Geometry check sheet. Reference: the model listing, model coordinates, mm. Face numbers are marked on the shaded views. A direction names the side the tool comes from. Give positions to 0.01 mm unless a question says otherwise; leave off trailing zeros. Write each loop counter-clockwise with the first axis right and the second up, starting at its lowest first coordinate (ties: lowest second). Pieces come first, ordered by that corner, then holes. Notation, with made-up numbers: (-29.75, 3) -> (-12.75, 3) arc R30 ccw to (-12.75, 41) -> close; hole circle Ø5 at (19.5, 58). An arc over 180 degrees is marked (long way). Write item = value, one per line. Start each with the question number.
1. Depth check by flat-ended pin: P1, Ø5, axis at x = 67, z = -4.5, coming from the -Y side; P2, Ø20, axis at x = 71.5, z = -2, coming from the +Y side; P3, Ø2, axis at y = 31.5, z = 40.5, coming from the +X side; P4, Ø4, axis at x = 70.03, z = -10, coming from the +Y side. Enter the tip coordinate at first touch or a pass-through.
2. Set-up check for the marked faces 1, 2 and 3: record each of +Z, -Z, +X, -X, +Y, -Y from which the full face is reachable in a straight line by a thin tool's end or side.
3. Cross-section at C-C, the plane y = 21. Record the cut outline in (x, z), plus the area to 3 significant figures.
4. Cross-section at A-A, the plane z = 41.5. Record the cut outline in (x, y).
5. Cross-section at D-D, the plane z = -10. State how many separate pieces and enclosed holes the cut face has, plus the area to 3 significant figures.
6. Thickness scan on line 1 along X through (y, z) = (9, -10); line 2 along Y through (x, z) = (40.75, 10.5); line 3 along Z through (x, y) = (40.5, 36.5). Record the ranges inside material, lowest first.
7. Mould release check, pull along Y, two halves, no side actions. Record for the marked faces 4, 5 and 6: pulls with the +Y half, pulls with the -Y half, needs draft (parallel to the pull), parting line crosses it, or undercut.
8. Cross-section at B-B, the plane x = 44. Record the cut outline in (y, z), plus the area to 3 significant figures.
```python
from build123d import *

# Parameters (mm, degrees)
SKETCH1_W           = 67
SKETCH1_H           = 41.999999434
BOSS_EXTRUDE1_DEPTH = 6.000000983
SKETCH2_W           = 24.999999441
SKETCH2_H           = 29.999998398
BOSS_EXTRUDE2_DEPTH = 50
SKETCH3_W           = 19.999999553
SKETCH3_H           = 19.999999553
CUT_EXTRUDE1_DEPTH  = 85.314886613
SKETCH14_R          = 11.2
CUT_EXTRUDE12_DEPTH = 10
SKETCH15_R          = 2.6
CUT_EXTRUDE13_DEPTH = 112.961295121
SKETCH18_R          = 1.5
CUT_EXTRUDE14_DEPTH = 81.454956308
SKETCH19_R          = 2.6
CUT_EXTRUDE15_DEPTH = 113.063962124
SKETCH20_R          = 28.543107088
BOSS_EXTRUDE3_DEPTH = 5
BOSS_EXTRUDE4_REACH = 132.242
SKETCH21_W          = 30.03647221
SKETCH21_H          = 5
SKETCH22_W          = 8.074560758
SKETCH22_H          = 29.943227156
CUT_EXTRUDE16_DEPTH = 10


with BuildPart() as part:
    # Sketch1 → Boss-Extrude1 (new body)
    with BuildSketch(Plane(origin=(45.028056949, 0, 0), x_dir=(0, 0, -1), z_dir=(1, 0, 0))):
        with Locations((-13.500000447, 20.999999717)):
            Rectangle(SKETCH1_W, SKETCH1_H)
    extrude(amount=-BOSS_EXTRUDE1_DEPTH)

    # Sketch2 → Boss-Extrude2 (add)
    with BuildSketch(Plane(origin=(45.028056949, 0, 0), x_dir=(0, 0, -1), z_dir=(1, 0, 0))):
        with Locations((7.499999833, 20.999999251)):
            Rectangle(SKETCH2_W, SKETCH2_H)
    extrude(amount=BOSS_EXTRUDE2_DEPTH)

    # Sketch3 → Cut-Extrude1 (cut, through all)
    with BuildSketch(Plane.ZY.offset(-39.028055966)):
        with Locations((-9.999999777, 20.999999716)):
            Rectangle(SKETCH3_W, SKETCH3_H)
    extrude(amount=-CUT_EXTRUDE1_DEPTH, mode=Mode.SUBTRACT)

    # Sketch14 → Cut-Extrude12 (cut)
    with BuildSketch(Plane(origin=(45.028056949, 0, 0), x_dir=(0, 0, -1), z_dir=(1, 0, 0))):
        with Locations((-25.999999888, 20.999999251)):
            Circle(SKETCH14_R)
    extrude(amount=-CUT_EXTRUDE12_DEPTH, mode=Mode.SUBTRACT)

    # Sketch15 → Cut-Extrude13 (cut, through all)
    with BuildSketch(Plane(origin=(0, 6.000000052, 0), x_dir=(-1, 0, 0), z_dir=(0, -1, 0))):
        with Locations(Location((-50.028056949, 9.999999553, 0), (0, 0, 90))):
            Circle(SKETCH15_R)
        with Locations(Location((-70.028056949, 9.999999553, 0), (0, 0, 90))):
            Circle(SKETCH15_R)
    extrude(amount=-CUT_EXTRUDE13_DEPTH, mode=Mode.SUBTRACT)

    # Sketch18 → Cut-Extrude14 (cut, through all)
    with BuildSketch(Plane(origin=(45.028056949, 0, 0), x_dir=(0, 0, -1), z_dir=(1, 0, 0))):
        with Locations((-10.499999888, 36.499999251)):
            Circle(SKETCH18_R)
        with Locations((-10.499999888, 5.499999251)):
            Circle(SKETCH18_R)
        with Locations((-41.499999888, 5.499999251)):
            Circle(SKETCH18_R)
        with Locations((-41.499999888, 36.499999251)):
            Circle(SKETCH18_R)
    extrude(amount=-CUT_EXTRUDE14_DEPTH, mode=Mode.SUBTRACT)

    # Sketch19 → Cut-Extrude15 (cut, through all)
    with BuildSketch(Plane.XY.offset(4.999999888)):
        with Locations((70.028056949, 20.999999251)):
            Circle(SKETCH19_R)
    extrude(amount=-CUT_EXTRUDE15_DEPTH, mode=Mode.SUBTRACT)

    # Sketch20 → Boss-Extrude3 (add)
    with BuildSketch(Plane(origin=(95.028056949, 0, 0), x_dir=(0, 0, -1), z_dir=(1, 0, 0))):
        with Locations(Location((-6.802134848, 21.140269153, 0), (0, 0, 327.965134835))):
            Circle(SKETCH20_R)
    extrude(amount=BOSS_EXTRUDE3_DEPTH)

    # Sketch21 → Boss-Extrude4 (add, up to next)
    with BuildSketch(Plane.YX.offset(19.999999553), mode=Mode.PRIVATE) as boss_extrude4_sk1:
        with Locations((21.018236157, 97.528056949)):
            Rectangle(SKETCH21_W, SKETCH21_H)
    boss_extrude4_tool1 = extrude(boss_extrude4_sk1.sketch, amount=-BOSS_EXTRUDE4_REACH, mode=Mode.PRIVATE) - part.part
    add(boss_extrude4_tool1.solids().sort_by_distance((97.528057, 21.018236, -20))[0])
    add(boss_extrude4_tool1.solids().sort_by_distance((97.528057, 21.018236, -20))[1])

    # Sketch22 → Cut-Extrude16 (cut)
    with BuildSketch(Plane(origin=(100.028056949, 0, 0), x_dir=(0, 0, -1), z_dir=(1, 0, 0))):
        with Locations((24.037279932, 20.970137181)):
            Rectangle(SKETCH22_W, SKETCH22_H)
    extrude(amount=-CUT_EXTRUDE16_DEPTH, mode=Mode.SUBTRACT)


solid = part.part
```
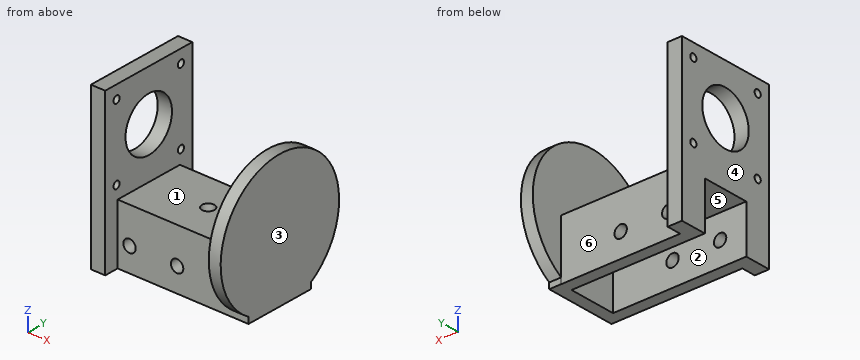
Answers:
q1.P1 = 6
q1.P2 = 36
q1.P3 = 45.03
q1.P4 = through
q2.face_1 = +Z, +Y, -Y
q2.face_2 = -Z, -X
q2.face_3 = +Z, -Z, +X, +Y, -Y
q3.outline = (39.03, 0) -> (67.43, 0) -> (67.43, 5) -> (45.03, 5) -> (45.03, 14.8) -> (39.03, 14.8) -> close; (39.03, 37.2) -> (45.03, 37.2) -> (45.03, 47) -> (39.03, 47) -> close; (72.63, 0) -> (95.03, 0) -> (95.03, -20) -> (100.03, -20) -> (100.03, 35.34) -> (95.03, 35.34) -> (95.03, 5) -> (72.63, 5) -> close
q3.area = 648 mm^2
q4.outline = (39.03, 0) -> (45.03, 0) -> (45.03, 4) -> (39.03, 4) -> close; (39.03, 7) -> (45.03, 7) -> (45.03, 35) -> (39.03, 35) -> close; (39.03, 38) -> (45.03, 38) -> (45.03, 42) -> (39.03, 42) -> close
q5.separate_pieces = 5
q5.enclosed_holes = 0
q5.area = 759 mm^2
q6.line_1 = 39.03 to 47.43, 52.63 to 67.43, 72.63 to 100.03
q6.line_2 = 0 to 4, 7 to 35, 38 to 42
q6.line_3 = -20 to 9, 12 to 40, 43 to 47
q7.face_4 = needs draft
q7.face_5 = undercut
q7.face_6 = pulls with the +Y half
q8.outline = (0, -20) -> (11, -20) -> (11, 0) -> (31, 0) -> (31, -20) -> (42, -20) -> (42, 47) -> (0, 47) -> close; hole circle Ø3 at (5.5, 10.5); hole circle Ø3 at (5.5, 41.5); hole circle Ø22.4 at (21, 26); hole circle Ø3 at (36.5, 10.5); hole circle Ø3 at (36.5, 41.5)
q8.area = 1,990 mm^2
